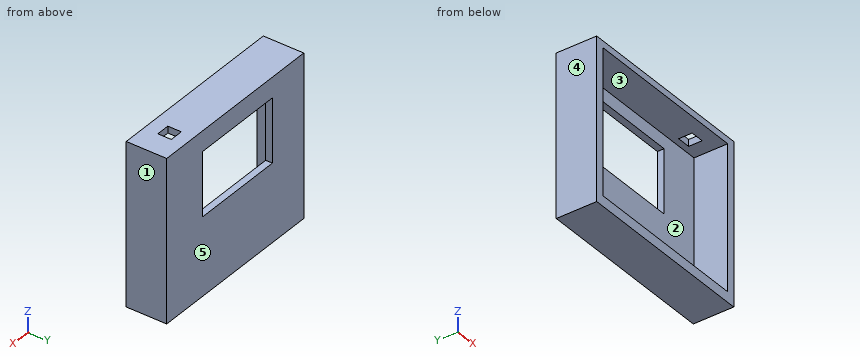
```python
from build123d import *

# Parameters (mm, degrees)
F0_W     = 69.85
F0_H     = 60.96
F1_DEPTH = 15.24
F2_W     = 63.5
F2_H     = 54.530626
F3_DEPTH = 12.7
F4_W     = 5.08
F4_H     = 5.08
F5_DEPTH = 25.4
F7_DEPTH = 25.4


with BuildPart() as f1:
    # F0 (on Front) → F1 (new body)
    with BuildSketch(Plane.XZ):
        with Locations((9.194272, -19.248438)):
            Rectangle(F0_W, F0_H)
    extrude(amount=F1_DEPTH)

    # F2 (on face) → F3 (cut)
    with BuildSketch(Plane.XZ.offset(15.24)):
        with Locations((9.300105, -18.573751)):
            Rectangle(F2_W, F2_H)
    extrude(amount=-F3_DEPTH, mode=Mode.SUBTRACT)

    # F4 (on face) → F5 (cut)
    with BuildSketch(Plane.XY.offset(11.231562)):
        with Locations((32.606527, -7.426056)):
            Rectangle(F4_W, F4_H)
    extrude(amount=-F5_DEPTH, mode=Mode.SUBTRACT)

    # F6 (on face) → F7 (cut)
    with BuildSketch(Plane.XZ.offset(2.54)):
        Polygon((-9.749895, 3.611562), (-9.749895, -11.760729), (-9.749895, -20.439064), (25.836561, -20.439064), (25.836561, 3.611562), (9.300105, 3.611562), align=None)
    extrude(amount=-F7_DEPTH, mode=Mode.SUBTRACT)


solid = f1.part
```
Design review of the part built by this model. Coordinates are the model's own, in mm. Face numbers are marked on the shaded views. A direction names the side the tool comes from. Coordinates: 2 decimals unless noted, no trailing zeros. Order: outer loops, then holes, each group sorted by start corner. A loop starts at its lowest first (then second) coordinate and runs counter-clockwise, first axis right, second up.
1) Take a section at B-B, the plane z = -11. Give the boundary of the cut face in (x, y).
2) Wall thickness on line 1 along X through (y, z) = (-4, -23.5); line 2 along Z through (x, y) = (29.5, -10.75); line 3 along X through (y, z) = (-0.25, 3): over which ranges is each line inside the solid? List them lowest first.
3) Mouldability with a two-part tool opening along X and no side actions: class the marked faces 3, 4 and 5 as +X half, -X half, draft (parallel to the pull), parting line (faces both ways), or undercut.
4) Take a section at C-C, the plane y = -6. Give the boundary of the cut face in (x, z), and give its area (3 significant figures).
5) For the marked faces 1 and 2, list the 3-axis set-ups (+Z, -Z, +X, -X, +Y, -Y) from which the entire face can be reached by the end or side of a thin tool; tool diameter is ignored.
6) Take a section at D-D, the plane y = -11.5. Give the boundary of the cut face in (x, z), and give its area (3 significant figures).
7) Take a section at A-A, the plane x = 17.5. Give the boundary of the cut face in (y, z), and give its area (3 significant figures).
Returned:
1. outline: (-25.73, -15.24) - (-22.45, -15.24) - (-22.45, -2.54) - (-9.75, -2.54) - (-9.75, 0) - (-25.73, 0) - close; (25.84, -2.54) - (41.05, -2.54) - (41.05, -15.24) - (44.12, -15.24) - (44.12, 0) - (25.84, 0) - close
2. line 1: x = -25.73 to -22.45, 41.05 to 44.12
2. line 2: z = -49.73 to -45.84, 8.69 to 11.23
2. line 3: x = -25.73 to -9.75, 25.84 to 44.12
3. face 3: undercut
3. face 4: -X half
3. face 5: draft
4. outline: (-25.73, -49.73) - (44.12, -49.73) - (44.12, 11.23) - (35.15, 11.23) - (35.15, 8.69) - (41.05, 8.69) - (41.05, -45.84) - (-22.45, -45.84) - (-22.45, 8.69) - (30.07, 8.69) - (30.07, 11.23) - (-25.73, 11.23) - close
4. area: 782 mm2
5. face 1: +Z, -Z, +X, +Y, -Y
5. face 2: -Y
6. outline: (-25.73, -49.73) - (44.12, -49.73) - (44.12, 11.23) - (-25.73, 11.23) - close; hole (-22.45, -45.84) - (41.05, -45.84) - (41.05, 8.69) - (-22.45, 8.69) - close
6. area: 795 mm2
7. outline: (-15.24, -49.73) - (0, -49.73) - (0, -20.44) - (-2.54, -20.44) - (-2.54, -45.84) - (-15.24, -45.84) - close; (-15.24, 8.69) - (-2.54, 8.69) - (-2.54, 3.61) - (0, 3.61) - (0, 11.23) - (-15.24, 11.23) - close
7. area: 175 mm2
